Build history of the part. All positions in model axes, mm. Face numbers are marked on the shaded views. A direction names the side the tool comes from. Coordinates: 2 decimals unless noted, no trailing zeros. Loops run counter-clockwise (first coordinate to the right, second up) from the corner with the lowest first, then second, coordinate; pieces in that order, holes last.
Item 1: Flat gauge pins, fed straight in: pin 1 (3.5 mm diameter, centred on y = -4, z = 10.5, fed in from +X); pin 2 (2 mm diameter, centred on x = 7.5, z = 5, fed in from +Y); pin 3 (3 mm diameter, centred on x = -16, y = -4, fed in from -Z). Where does each tip first touch, or does it go through?
Item 2: Drill centre lines: line 1 along Z through (x, y) = (-12.75, -4); line 2 along Z through (x, y) = (-15, -4); line 3 along Z through (x, y) = (-12.5, -17.5). Where is each one in solid material? Low to high.
Item 3: Cut at A-A (z = 6). List the corners of the cut face in (x, y) (3 decimals).
Item 4: Cut at B-B (y = -36). List the corners of the cut face in (x, z).
Item 5: 3-axis set-ups, long thin cutter, end or side, ignore diameter. For the marked faces 1, 2, 3 and 4: which of +Z, -Z, +X, -X, +Y, -Y reach the whole face in a straight line?
Item 6: Mould opens along Y. For the marked faces 5, 6 and 7 say: released by +Y, released by -Y, zero draft, split by the parting line, or undercut.
Item 7: Cut at C-C (y = 11.5). List the corners of the cut face in (x, z), and give its area (3 significant figures).
Item 8: Cut at D-D (y = -26.5). List the corners of the cut face in (x, z), and give its area (4 significant figures).
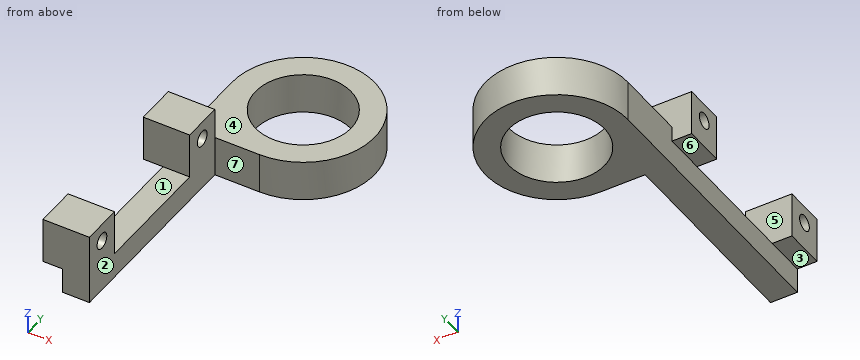
from build123d import *

# Parameters (mm, degrees)
F0_R     = 9.375
F1_DEPTH = 8
F2_W     = 5.25
F2_H     = 40
F3_DEPTH = 5
F5_DEPTH = 9
F7_D     = 3.1


with BuildPart() as f1:
    # F0 (on Top) → F1 (new body)
    with BuildSketch(Plane.XY):
        with BuildLine():
            Line((-14, 0), (0, 0))
            ThreePointArc((0, 0), (9.899495, 23.899495), (-14, 14))
            Line((-14, 14), (-14, 0))
        make_face()
        with Locations((0, 14)):
            Circle(F0_R, mode=Mode.SUBTRACT)
    extrude(amount=F1_DEPTH)

    # F2 (on Top) → F3 (join)
    with BuildSketch(Plane.XY):
        with Locations((-11.375, -20)):
            Rectangle(F2_W, F2_H)
    extrude(amount=F3_DEPTH)

    # F4 (on face) → F5 (join)
    with BuildSketch(Plane.XY.offset(5)):
        Polygon((-8.75, -40), (-8.75, -32), (-17.85, -32), (-17.85, -40), (-14, -40), align=None)
        Polygon((-8.75, 0), (-14, 0), (-17.85, 0), (-17.85, -8), (-8.75, -8), align=None)
    extrude(amount=F5_DEPTH)

    # F7 (through all)
    with Locations(Plane(origin=(-17.85, 0, 0), x_dir=(0, -1, 0), z_dir=(-1, 0, 0))):
        with Locations((4, 10.5), (36, 10.5)):
            Hole(F7_D / 2)


solid = f1.part
Filled sheet:
1. pin 1: stops at x = -8.75
1. pin 2: stops at y = 26.4
1. pin 3: stops at z = 5
2. line 1: z = 0 to 8.95, 12.05 to 14
2. line 2: z = 5 to 8.95, 12.05 to 14
2. line 3: z = 0 to 5
3. outline: (-17.85, -40) - (-8.75, -40) - (-8.75, -32) - (-17.85, -32) - close; (-17.85, -8) - (-8.75, -8) - (-8.75, 0) - (0, 0) arc R14 ccw (long way) to (-14, 14) - (-14, 0) - (-17.85, 0) - close; hole circle Ø18.75 at (0, 14)
4. outline: (-17.85, 5) - (-14, 5) - (-14, 0) - (-8.75, 0) - (-8.75, 8.95) - (-17.85, 8.95) - close; (-17.85, 12.05) - (-8.75, 12.05) - (-8.75, 14) - (-17.85, 14) - close
5. face 1: +Z, +X, -X
5. face 2: +Z, -Z, +X, -Y
5. face 3: -Z, -X, +Y, -Y
5. face 4: +Z, +X, -X, +Y
6. face 5: undercut
6. face 6: zero draft
6. face 7: released by -Y
7. outline: (-14, 0) - (-9.04, 0) - (-9.04, 8) - (-14, 8) - close; (9.04, 0) - (13.77, 0) - (13.77, 8) - (9.04, 8) - close
7. area: 77.6 mm2
8. outline: (-14, 0) - (-8.75, 0) - (-8.75, 5) - (-14, 5) - close
8. area: 26.25 mm2
